Autodesk Inventor part; units mm, degrees
ref_plane "Work Plane1" through (-17.4436, 0, 0) normal (0, -0.866, -0.5) x (1, 0, 0)
ref_plane "YZ Plane" through (0, 0, 0) normal (1, 0, 0) x (0, 1, 0)
ref_plane "XZ Plane" through (0, 0, 0) normal (0, 1, 0) x (-1, 0, 0)
sketch "Sketch1" plane through (0, 0, 0) normal (1, 0, 0) x (0, 1, 0)
  line L0 (-9.2376, 0) -> (-4.6188, 8)
  line L1 (-4.6188, 8) -> (4.6188, 8)
  line L2 (4.6188, 8) -> (9.2376, 0)
  line L3 (9.2376, 0) -> (4.6188, -8)
  line L4 (4.6188, -8) -> (-4.6188, -8)
  line L5 (-4.6188, -8) -> (-9.2376, 0)
  point P0 (0, 0)
  point P1 (0, 0)
  dimension "d0" = 18.4752
extrude "Body" add sketch "Sketch1" along normal blind 8.4
sketch "Sketch2" plane through (0, 0, 0) normal (0, 0, 1) x (1, 0, 0)
  line L0 (0, 4.6188) -> (0, 9.2376)
  line L1 (0, 9.2376) -> (8.4, 9.2376)
  line L2 (8.4, 4.6188) -> (8.4, 9.2376)
  line L3 (-1.68, 0) -> (10.08, 0)
  line L4 (0.7145, 9.2376) -> (0, 8)
  line L5 (7.6855, 9.2376) -> (8.4, 8)
  dimension "d3" = 30
  dimension "d4" = 30
  dimension "d5" = 16
  dimension "d6" = 16
revolve "Chamfer1" cut sketch "Sketch2" angle 360 about axis through (-10, 0, 0) along (1, 0, 0)
sketch "Sketch3" plane through (8.4, 0, 0) normal (1, 0, 0) x (0, 0, -1)
  arc A0 (-4, -6.9282) -> (4, -6.9282) centre (0, 0) ccw
hole "Thread" at (8.4, 0, 0) direction (-1, 0, 0) diameter 8.376 end through all
chamfer "Chamfer2" distance 0.8119 angle 30 1 edges at (8.4, 0, 4.188) measured on face at (8.4, -6.6899, -0.1683)
chamfer "Chamfer3" distance 0.8119 angle 30 1 edges at (0, 0, 4.188) measured on face at (0, -6.6899, -0.1683)
ref_plane "Work Plane1" through (-17.4436, 0, 0) normal (0, -0.866, -0.5) x (1, 0, 0)
equation "\"d0\" = 1.1547 * SW"
equation "\"d1\" = KOH"
equation "\"d8\" = -0.5 * GD1 + 0.5 * NND"
equation "\"d40\" = -0.5 * GD1 + 0.5 * NND"
equation "\"d10\" = -0.5 * GD1 + 0.5 * NND"
equation "\"d41\" = -0.5 * GD1 + 0.5 * NND"
equation "\"d3\" = ANG1"
equation "\"d4\" = ANG2"
equation "\"d5\" = SW0"
equation "\"d6\" = SW01"
equation "\"ANG1\" = 30deg"
equation "\"ANG2\" = 30deg"
equation "\"KOH\" = 8.4"
equation "\"SW\" = 16"
equation "\"SW0\" = SW"
equation "\"SW01\" = SW"
equation "\"GUL\" = 0.541266 * PTC"
equation "\"WFT\" = 0.6"
equation "\"TOA\" = 30deg"
equation "\"PTC\" = 1.5"
equation "\"E0\" = 1.155 * SW"
equation "\"GAL\" = 0.541266 * PTC"
properties part number "AS 1112 - M10  Type 5" material "Steel, Mild"
For this review, take the finished solid that the model builds, in its own axes (mm). Coordinates: 2 decimals unless noted, no trailing zeros. Order: outer loops, then holes, each group sorted by start corner. A loop starts at its lowest first (then second) coordinate and runs counter-clockwise, first axis right, second up. Notation, with made-up numbers: (36, 30) - (60, 30) arc R29 ccw to (60, 50) - close; hole circle Ø2 at (2, 26.5). An arc over 180 degrees is marked (long way). Answer as a JSON object with one key per item and string values. Group by question number.
1. For probe 1 along Z at (x, y) = (5.5, 0); probe 2 along Y at (x, z) = (2.75, 3.5); probe 3 along Y at (x, z) = (6.25, 3.75), list the stretches that pass through material, from the lowest coordinate up.
2. We need section A-A on x = 3. State the section outline as (y, z) points, then the cut area to 3 significant figures.
3. The part is to be moulded in two halves that separate along Y. For faces 1 (the cylindrical face through (4.148, -2.83, 3.087)), 2 (the flat face through (4, 0, -8)), 3 (the conical face through (0.174, 8.301, -0.02)), say which applies: pulls with the +Y half, pulls with the -Y half, needs draft (parallel to the pull), parting line crosses it, or undercut.
Final values:
{
 "1": {"probe 1": "-8 to -4.19, 4.19 to 8", "probe 2": "-7.22 to -2.3, 2.3 to 7.22", "probe 3": "-7.07 to -1.86, 1.86 to 7.07"},
 "2": {"outline": "(-9.24, 0) - (-4.62, -8) - (4.62, -8) - (9.24, 0) - (4.62, 8) - (-4.62, 8) - close; hole circle Ø8.38 at (0, 0)", "area": "167 mm²"},
 "3": {"face 1": "undercut", "face 2": "needs draft", "face 3": "pulls with the +Y half"}
}
